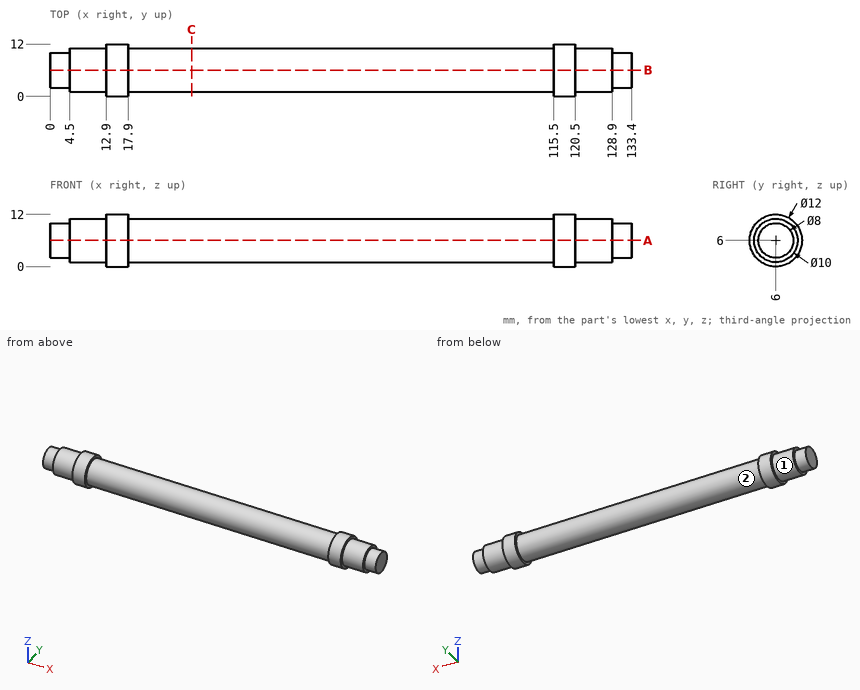
Verification items for this drawing (mm, ordinates from the low corner). Round coordinates to 2 decimals unless told otherwise and drop trailing zeros. Write each loop counter-clockwise with the first axis right and the second up, starting at its lowest first coordinate (ties: lowest second). Pieces come first, ordered by that corner, then holes. Notation, with made-up numbers: (19, 51) - (36, 51) arc R18 ccw to (36, 69) - close; hole circle Ø11 at (-15, 67). An arc over 180 degrees is marked (long way). Answer as a JSON object with one key per item and string values. Group by question number.
Q1. Section check A-A, the plane z = 6. Enter the section's corners in (x, y).
Q2. Section check C-C, the plane x = 32.5. Enter the section's corners in (y, z).
Q3. Mould release check, pull along X, two halves, no side actions. Record for the marked faces 1 and 2: released by +X, released by -X, zero draft, split by the parting line, or undercut.
Q4. Go/stop test with flat-tipped pins: pin 1 Ø6 at (x, y) = (34.5, 2) entering from +Z; pin 2 Ø2 at (x, y) = (35.5, 7.5) entering from +Z; pin 3 Ø6 at (x, z) = (20.5, 3) entering from -Y. Record where each tip stops, or that it passes through.
Q5. Thickness scan on line 1 (X direction, y = 5.5, z = 0.5); line 2 (Z direction, x = 52.5, y = 5.5); line 3 (Z direction, x = 23.5, y = 3). Record the ranges inside material, lowest first.
Found:
{
 "1": {"outline": "(0, 2) - (4.5, 2) - (4.5, 1) - (12.9, 1) - (12.9, 0) - (17.9, 0) - (17.9, 1) - (115.5, 1) - (115.5, 0) - (120.5, 0) - (120.5, 1) - (128.9, 1) - (128.9, 2) - (133.4, 2) - (133.4, 10) - (128.9, 10) - (128.9, 11) - (120.5, 11) - (120.5, 12) - (115.5, 12) - (115.5, 11) - (17.9, 11) - (17.9, 12) - (12.9, 12) - (12.9, 11) - (4.5, 11) - (4.5, 10) - (0, 10) - close"},
 "2": {"outline": "circle Ø10 at (6, 6)"},
 "3": {"face 1": "zero draft", "face 2": "undercut"},
 "4": {"pin 1": "stops at z = 10.9", "pin 2": "stops at z = 10.97", "pin 3": "stops at y = 0.19"},
 "5": {"line 1": "x = 12.9 to 17.9, 115.5 to 120.5", "line 2": "z = 1.03 to 10.97", "line 3": "z = 2 to 10"}
}
